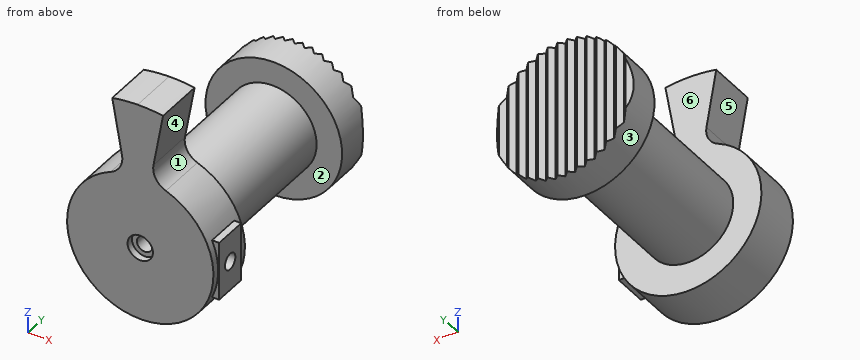
from build123d import *

# Parameters (mm, degrees)
SKETCH1_R                = 7.5
BOSS_EXTRUDE1_DEPTH      = 5
SKETCH2_R                = 7
BOSS_EXTRUDE2_DEPTH      = 20
CUT_EXTRUDE2_DEPTH       = 28.156951228
CUT_EXTRUDE2_DEPTH_BACK  = 28.156951228
SKETCH6_R                = 1.3
CUT_EXTRUDE3_DEPTH       = 0.7
SKETCH9_R                = 0.8
CUT_EXTRUDE4_DEPTH       = 7
BOSS_EXTRUDE3_DEPTH      = 0.1
BOSS_EXTRUDE3_DEPTH_BACK = 1
SKETCH10_W               = 6
SKETCH10_H               = 3.5
SKETCH17_R               = 7.5
SKETCH17_R_2             = 4.5
CUT_EXTRUDE7_DEPTH       = 16.2
BOSS_EXTRUDE6_DEPTH      = 5
FILLET2_R                = 2
SKETCH11_R               = 0.825
CUT_EXTRUDE8_DEPTH       = 7.5


with BuildPart() as part:
    # Sketch1 → Boss-Extrude1 (new body)
    with BuildSketch(Plane(origin=(0, 0, 0), x_dir=(1, 0, 0), z_dir=(0, 1, 0))):
        with Locations(Location((0, 0, 0), (0, 0, 270))):
            Circle(SKETCH1_R)
    extrude(amount=BOSS_EXTRUDE1_DEPTH)

    # Sketch2 → Boss-Extrude2 (add)
    with BuildSketch(Plane(origin=(0, 5, 0), x_dir=(1, 0, 0), z_dir=(0, 1, 0))):
        with Locations(Location((0, 0, 0), (0, 0, 270))):
            Circle(SKETCH2_R)
    extrude(amount=BOSS_EXTRUDE2_DEPTH)

    # Sketch5 → Cut-Extrude2 (cut, two sides: drawn at the far end of the back side and taken through both)
    with BuildSketch(Plane.XY.offset(-CUT_EXTRUDE2_DEPTH_BACK)):
        Polygon((-7.502045815, 25), (-7, 24.497954185), (-6.502045815, 25), (-6, 24.497954185), (-5.502045815, 25), (-5, 24.497954185), (-4.502045815, 25), (-4, 24.497954185), (-3.502045815, 25), (-3, 24.497954185), (-2.502045815, 25), (-2, 24.497954185), (-1.502045815, 25), (-1, 24.497954185), (-0.502045815, 25), (0, 24.497954185), (0.497954185, 25), (1, 24.497954185), (1.497954185, 25), (2, 24.497954185), (2.497954185, 25), (3, 24.497954185), (3.497954185, 25), (4, 24.497954185), (4.497954185, 25), (5, 24.497954185), (5.497954185, 25), (6, 24.497954185), (6.497954185, 25), (7, 24.497954185), (7, 25.505612795), (-7.502045815, 25.505612795), align=None)
    extrude(amount=CUT_EXTRUDE2_DEPTH + CUT_EXTRUDE2_DEPTH_BACK, mode=Mode.SUBTRACT)

    # Sketch6 → Cut-Extrude3 (cut)
    with BuildSketch(Plane.XZ):
        with Locations(Location((0, 0, 0), (0, 0, 270))):
            Circle(SKETCH6_R)
    extrude(amount=-CUT_EXTRUDE3_DEPTH, mode=Mode.SUBTRACT)

    # Sketch9 → Cut-Extrude4 (cut)
    with BuildSketch(Plane.XZ.offset(-0.7)):
        with Locations(Location((0, 0, 0), (0, 0, 270))):
            Circle(SKETCH9_R)
    extrude(amount=-CUT_EXTRUDE4_DEPTH, mode=Mode.SUBTRACT)

    # Sketch10 → Boss-Extrude3 (add, two sides: drawn at the far end of the back side and taken through both)
    with BuildSketch(Plane(origin=(7.5, 0, 0), x_dir=(0, 0, -1), z_dir=(1, 0, 0)).offset(-BOSS_EXTRUDE3_DEPTH_BACK)):
        with Locations((0, 2.5)):
            Rectangle(SKETCH10_W, SKETCH10_H)
    extrude(amount=BOSS_EXTRUDE3_DEPTH + BOSS_EXTRUDE3_DEPTH_BACK)

    # Sketch17 → Cut-Extrude7 (cut)
    with BuildSketch(Plane(origin=(0, 5, 0), x_dir=(1, 0, 0), z_dir=(0, 1, 0))):
        with Locations(Location((0, 0, 0), (0, 0, 270))):
            Circle(SKETCH17_R)
        with Locations(Location((-0.11397387, 0, 0), (0, 0, 270))):
            Circle(SKETCH17_R_2, mode=Mode.SUBTRACT)
    extrude(amount=CUT_EXTRUDE7_DEPTH, mode=Mode.SUBTRACT)

    # Sketch20 → Boss-Extrude6 (add)
    with BuildSketch(Plane.XZ):
        with BuildLine():
            Line((0.70668366, 5.570291045), (2.337095188, 14.816814303))
            ThreePointArc((2.337095188, 14.816814303), (1.03683138, 14.964123118), (-0.271323341, 14.997545921))
            ThreePointArc((-0.271323341, 14.997545921), (-1.577413128, 14.916828343), (-2.871497849, 14.722584695))
            Line((-2.871497849, 14.722584695), (-1.241086321, 5.476061437))
            ThreePointArc((-1.241086321, 5.476061437), (-0.759093411, 5.56339117), (-0.271323341, 5.608380137))
            ThreePointArc((-0.271323341, 5.608380137), (0.218511662, 5.610685945), (0.70668366, 5.570291045))
        make_face()
    extrude(amount=-BOSS_EXTRUDE6_DEPTH)

    # Fillet2
    fillet2_edges = [part.edges().sort_by_distance(p)[0] for p in [
        (1.0343075, 2.5, 7.428338172),
        (-1.568710161, 2.5, 7.334108564),
    ]]
    fillet(fillet2_edges, radius=FILLET2_R)

    # Sketch11 → Cut-Extrude8 (cut)
    with BuildSketch(Plane(origin=(7.6, 0, 0), x_dir=(0, 0, -1), z_dir=(1, 0, 0))):
        with Locations((0, 2.5)):
            Circle(SKETCH11_R)
    extrude(amount=-CUT_EXTRUDE8_DEPTH, mode=Mode.SUBTRACT)


solid = part.part
Design review of the part built by this model. Coordinates are the model's own, in mm. Face numbers are marked on the shaded views. A direction names the side the tool comes from. Coordinates: 2 decimals unless noted, no trailing zeros. Order: outer loops, then holes, each group sorted by start corner. A loop starts at its lowest first (then second) coordinate and runs counter-clockwise, first axis right, second up.
Item 1: Take a section at A-A, the plane y = 23.25. Write out the cut boundary in (x, z).
Item 2: For line 1 (X direction, y = 0.4, z = 0); line 2 (X direction, y = 6.25, z = 0); line 3 (Y direction, x = 6.25, z = 0) (3 decimals), list the stretches that pass through material, from the lowest coordinate up.
Item 3: For pin 1 Ø6 at (x, y) = (6, 15) entering from +Z; pin 2 Ø4 at (y, z) = (16.5, -4) entering from +X; pin 3 Ø2 at (x, y) = (3, 18) entering from +Z, all flat-tipped, find the tip position at first contact; note any pin that passes through.
Item 4: The part is to be moulded in two halves that separate along Z. For the marked faces 3, 4, 5 and 6, say which applies: pulls with the +Z half, pulls with the -Z half, needs draft (parallel to the pull), parting line crosses it, or undercut.
Item 5: For the marked faces 1 and 2, list the 3-axis set-ups (+Z, -Z, +X, -X, +Y, -Y) from which the entire face can be reached by the end or side of a thin tool; tool diameter is ignored.
Item 6: Take a section at B-B, the plane z = 13.75. Write out the cut boundary in (x, y), then the cut area to 3 significant figures.
Item 7: Take a section at C-C, the plane y = 15. Write out the cut boundary in (x, z), then the cut area to 3 significant figures.
The answers:
1. outline: circle Ø14 at (0, 0)
2. line 1: x = -7.5 to -1.3, 1.3 to 7.5
2. line 2: x = -4.61 to -0.8, 0.8 to 4.39
2. line 3: y = 0 to 1.675, 3.325 to 5, 21.2 to 24.75
3. pin 1: stops at z = 3.25
3. pin 2: stops at x = 3.92
3. pin 3: stops at z = 3.97
4. face 3: parting line crosses it
4. face 4: undercut
4. face 5: undercut
4. face 6: needs draft
5. face 1: +X, +Y, -Y
5. face 2: none
6. outline: (-2.7, 0) - (2.15, 0) - (2.15, 5) - (-2.7, 5) - close
6. area: 24.2 mm2
7. outline: circle Ø9 at (-0.11, 0)
7. area: 63.6 mm2
